from build123d import *

# Parameters (mm, degrees)
SKETCH2_R           = 3.429
BOSS_EXTRUDE1_DEPTH = 12.7


with BuildPart() as part:
    # Sketch2 → Boss-Extrude1 (new body)
    with BuildSketch(Plane.XY):
        with BuildLine():
            Line((-10.840128061, -16.100640303), (-4.490128061, -22.450640303))
            ThreePointArc((-4.490128061, -22.450640303), (0, -24.310512242), (4.490128061, -22.450640303))
            Line((4.490128061, -22.450640303), (22.450640303, -4.490128061))
            ThreePointArc((22.450640303, -4.490128061), (24.310512242, 0), (22.450640303, 4.490128061))
            Line((22.450640303, 4.490128061), (16.100640303, 10.840128061))
            ThreePointArc((16.100640303, 10.840128061), (14.040552038, 12.216635031), (11.610512242, 12.7))
            Line((11.610512242, 12.7), (-6.35, 12.7))
            ThreePointArc((-6.35, 12.7), (-10.840128061, 10.840128061), (-12.7, 6.35))
            Line((-12.7, 6.35), (-12.7, -11.610512242))
            ThreePointArc((-12.7, -11.610512242), (-12.216635031, -14.040552038), (-10.840128061, -16.100640303))
        make_face()
        with Locations((15.875, 0)):
            Circle(SKETCH2_R, mode=Mode.SUBTRACT)
        with Locations((0, -15.875)):
            Circle(SKETCH2_R, mode=Mode.SUBTRACT)
        Polygon((6.35, 3.666174209), (0, 7.332348419), (-6.35, 3.666174209), (-6.35, -3.666174209), (0, -7.332348419), (6.35, -3.666174209), align=None, mode=Mode.SUBTRACT)
    extrude(amount=BOSS_EXTRUDE1_DEPTH)


solid = part.part
The model under review builds one solid part; all positions refer to its coordinate system, in mm. A direction names the side the tool comes from. Round coordinates to 2 decimals unless told otherwise and drop trailing zeros. Loops run counter-clockwise (first coordinate to the right, second up) from the corner with the lowest first, then second, coordinate; pieces in that order, holes last. Notation, with made-up numbers: M -1.5,34 L 17.5,34 A19 cw 17.5,39 Z; hole C 88.25,26 d5. An arc over 180 degrees is marked long. Answer as CSV lines item,"result".
1. We need section D-D (x = -7.5). Give the boundary of the cut face in (y, z) (3 decimals).
Outcome:
outline,"M -19.441,0 L 12.595,0 L 12.595,12.7 L -19.441,12.7 Z"
2. We need section A-A (y = 0). Give the boundary of the cut face in (x, z), plus the area to 3 significant figures.
Outcome:
outline,"M -12.7,0 L -6.35,0 L -6.35,12.7 L -12.7,12.7 Z; M 6.35,0 L 12.45,0 L 12.45,12.7 L 6.35,12.7 Z; M 19.3,0 L 24.31,0 L 24.31,12.7 L 19.3,12.7 Z"
area,"222 mm2"
3. For faces 1 (the face through (19.32, 7.62, 6.26)), 2 (the face through (-3.131, 5.525, 6.261)), list the 3-axis set-ups (+Z, -Z, +X, -X, +Y, -Y) from which the entire face can be reached by the end or side of a thin tool; tool diameter is ignored.
Outcome:
face 1,"+Z, -Z, +X, +Y"
face 2,"+Z, -Z"
4. Draft analysis for pull direction Y (two halves, no side actions). For faces 3 (the face through (24.31, -0.07, 6.26)), 4 (the face through (-6.35, 0, 6)), 5 (the face through (3, 12.7, 6)), state which applies: pulls with the +Y half, pulls with the -Y half, needs draft (parallel to the pull), parting line crosses it, or undercut.
Outcome:
face 3,"parting line crosses it"
face 4,"undercut"
face 5,"pulls with the +Y half"
5. To check wall thickness, follow L1, parallel to Y at x = 0, z = 3.5; L2, parallel to X at y = 0.5, z = 11.5; L3, parallel to Y at x = 1.5, z = 1. State the ranges of each line that lie inside material, in increasing order. Write a range as [from, to].
Outcome:
L1,"y = [-24.31, -19.3], [-12.45, -7.33], [7.33, 12.7]"
L2,"x = [-12.7, -6.35], [6.35, 12.48], [19.27, 24.29]"
L3,"y = [-24.13, -18.96], [-12.79, -6.47], [6.47, 12.7]"
6. We need section B-B (y = -15). Give the boundary of the cut face in (x, z), plus the area to 3 significant figures.
Outcome:
outline,"M -11.72,0 L -3.32,0 L -3.32,12.7 L -11.72,12.7 Z; M 3.32,0 L 11.94,0 L 11.94,12.7 L 3.32,12.7 Z"
area,"216 mm2"
7. We need section C-C (z = 11.25). Give the boundary of the cut face in (x, y) (3 decimals).
Outcome:
outline,"M -12.7,-11.611 A6.35 ccw -10.84,-16.101 L -4.49,-22.451 A6.35 ccw 4.49,-22.451 L 22.451,-4.49 A6.35 ccw 22.451,4.49 L 16.101,10.84 A6.35 ccw 11.611,12.7 L -6.35,12.7 A6.35 ccw -12.7,6.35 Z; hole M -6.35,-3.666 L 0,-7.332 L 6.35,-3.666 L 6.35,3.666 L 0,7.332 L -6.35,3.666 Z; hole C 0,-15.875 d6.858; hole C 15.875,0 d6.858"
8. Insertion check: pin 1 Ø12 at (x, y) = (-6, 1) entering from -Z; pin 2 Ø5 at (x, z) = (12, 7.5) entering from -Y. Each pin has a flat end and moves straight along its axis. Give the tip position at first contact, or say it passes through.
Outcome:
pin 1,"stops at z = 0"
pin 2,"stops at y = -17.44"
